Can you work these out from the model? Positions are in its coordinate system, mm. Face numbers are marked on the shaded views. A direction names the side the tool comes from. Give positions to 0.01 mm unless a question says otherwise; leave off trailing zeros. Order: outer loops, then holes, each group sorted by start corner. A loop starts at its lowest first (then second) coordinate and runs counter-clockwise, first axis right, second up. Notation, with made-up numbers: (73, 78) -> (119, 78) arc R10 cw to (119, 95) -> close; hole circle Ø11 at (43.25, -37.75). An arc over 180 degrees is marked (long way). Answer as a JSON object with one key per item and string values.
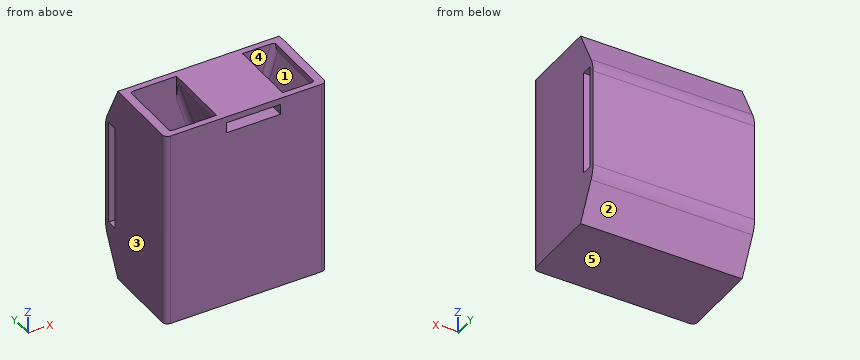
```python
from build123d import *

# Parameters (mm, degrees)
F1_DEPTH  = 3
F2_START  = 3
F2_DEPTH  = 32
F3_START  = 35
F3_DEPTH  = 3
F4_W      = 5
F4_H      = 50
F5_DEPTH  = 76.5907008807
F6_R      = 15
F8_R      = 2.5
F9_R      = 2.5
F7_W      = 25.5907008807
F7_H      = 5
F10_DEPTH = 35


with BuildPart() as f1:
    # F0 (on Front) → F1 (new body)
    with BuildSketch(Plane.XZ):
        Polygon((-29.1335783188, 93.8650974194), (0, 0), (18.3235442432, 0), (47.457122562, 93.8650974194), (43.384812198, 93.8650974194), (43.384812198, 90.8650974194), (16.1134965809, 3), (0.9311313508, 3), (28.2024469679, 90.8650974194), (28.2024469679, 93.8650974194), (-3.0730148629, 93.8650974194), (-3.0730148629, 90.8650974194), (10.9941265459, 45.5423573046), (0, 10.1205238455), (-25.0612679548, 90.8650974194), (-25.0612679548, 93.8650974194), align=None)
        Polygon((-3.0730148629, 93.8650974194), (-25.0612679548, 93.8650974194), (-25.0612679548, 90.8650974194), (0, 10.1205238455), (10.9941265459, 45.5423573046), (-3.0730148629, 90.8650974194), align=None)
        Polygon((43.384812198, 90.8650974194), (43.384812198, 93.8650974194), (28.2024469679, 93.8650974194), (28.2024469679, 90.8650974194), (0.9311313508, 3), (16.1134965809, 3), align=None)
        Polygon((-29.1335783188, 0), (0, 0), (-29.1335783188, 93.8650974194), align=None)
        Polygon((47.457122562, 93.8650974194), (18.3235442432, 0), (47.457122562, 0), align=None)
    extrude(amount=F1_DEPTH)

    # F0 (on Front) → F2 (join)
    with BuildSketch(Plane.XZ.offset(F2_START)):
        Polygon((-29.1335783188, 93.8650974194), (0, 0), (18.3235442432, 0), (47.457122562, 93.8650974194), (43.384812198, 93.8650974194), (43.384812198, 90.8650974194), (16.1134965809, 3), (0.9311313508, 3), (28.2024469679, 90.8650974194), (28.2024469679, 93.8650974194), (-3.0730148629, 93.8650974194), (-3.0730148629, 90.8650974194), (10.9941265459, 45.5423573046), (0, 10.1205238455), (-25.0612679548, 90.8650974194), (-25.0612679548, 93.8650974194), align=None)
        Polygon((-29.1335783188, 0), (0, 0), (-29.1335783188, 93.8650974194), align=None)
        Polygon((47.457122562, 93.8650974194), (18.3235442432, 0), (47.457122562, 0), align=None)
    extrude(amount=F2_DEPTH)

    # F0 (on Front) → F3 (join)
    with BuildSketch(Plane.XZ.offset(F3_START)):
        Polygon((-29.1335783188, 93.8650974194), (0, 0), (18.3235442432, 0), (47.457122562, 93.8650974194), (43.384812198, 93.8650974194), (43.384812198, 90.8650974194), (16.1134965809, 3), (0.9311313508, 3), (28.2024469679, 90.8650974194), (28.2024469679, 93.8650974194), (-3.0730148629, 93.8650974194), (-3.0730148629, 90.8650974194), (10.9941265459, 45.5423573046), (0, 10.1205238455), (-25.0612679548, 90.8650974194), (-25.0612679548, 93.8650974194), align=None)
        Polygon((-3.0730148629, 93.8650974194), (-25.0612679548, 93.8650974194), (-25.0612679548, 90.8650974194), (0, 10.1205238455), (10.9941265459, 45.5423573046), (-3.0730148629, 90.8650974194), align=None)
        Polygon((43.384812198, 90.8650974194), (43.384812198, 93.8650974194), (28.2024469679, 93.8650974194), (28.2024469679, 90.8650974194), (0.9311313508, 3), (16.1134965809, 3), align=None)
        Polygon((-29.1335783188, 0), (0, 0), (-29.1335783188, 93.8650974194), align=None)
        Polygon((47.457122562, 93.8650974194), (18.3235442432, 0), (47.457122562, 0), align=None)
    extrude(amount=F3_DEPTH)

    # F4 (on face) → F5 (join, through all)
    with BuildSketch(Plane.YZ.offset(47.457122562)):
        Polygon((10, 73.8650974194), (0, 93.8650974194), (0, 0), (10, 20), align=None)
        with Locations((5, 48.8650974194)):
            Rectangle(F4_W, F4_H, mode=Mode.SUBTRACT)
    extrude(amount=-F5_DEPTH)

    # F6
    f6_edges = [f1.edges().sort_by_distance(p)[0] for p in [
        (9.161772, 10, 73.865097),
        (9.161772, 10, 20),
    ]]
    fillet(f6_edges, radius=F6_R)

    # F8
    f8_edges = [f1.edges().sort_by_distance(p)[0] for p in [
        (-12.530634, -3, 50.492811),
        (3.960556, -3, 68.203727),
        (3.960556, -35, 68.203727),
        (-12.530634, -35, 50.492811),
        (29.749154, -35, 46.932549),
        (29.749154, -3, 46.932549),
        (14.566789, -3, 46.932549),
        (14.566789, -35, 46.932549),
    ]]
    fillet(f8_edges, radius=F8_R)

    # F9
    f9_edges = [f1.edges().sort_by_distance(p)[0] for p in [
        (-29.133578, -38, 46.932549),
        (47.457123, -38, 46.932549),
    ]]
    fillet(f9_edges, radius=F9_R)

    # F7 (on face) → F10 (cut)
    with BuildSketch(Plane.XZ.offset(38)):
        with Locations((12.6617721216, 88.3650974194)):
            Rectangle(F7_W, F7_H)
    extrude(amount=-F10_DEPTH, mode=Mode.SUBTRACT)


solid = f1.part
```
1. If we mould it in two halves opening along Z, with no side actions, what happens to the marked faces 1, 2 and 3? For each: +Z half, -Z half, draft (parallel to the pull), parting line (faces both ways), or undercut.
Worked answers:
{"face 1": "undercut", "face 2": "-Z half", "face 3": "draft"}
2. If we section it at C-C on z = 72.5: Count the separate pieces of the cut face and the enclosed holes in it, then the cut area to 3 significant figures.
Worked answers:
{"separate pieces": "2", "enclosed holes": "2", "area": "2,100 mm²"}
3. Will these pins go through, and if not, where does the flat tip stop? pin 1 Ø8 at (x, z) = (29.5, 15) entering from +Y; pin 2 Ø1.5 at (x, z) = (9.5, 89) entering from -Y; pin 3 Ø5.5 at (x, y) = (-2.5, 5) entering from +Z.
Worked answers:
{"pin 1": "y = 9.3", "pin 2": "y = -3", "pin 3": "z = 89.37"}
4. Please list where these lines run through material, in increasing order: L1, parallel to Y at x = 1.5, z = 38; L2, parallel to X at y = -34, z = 22; L3, parallel to X at y = -27, z = 20.
Worked answers:
{"L1": "-38 to -35, -3 to 2.5, 7.5 to 10", "L2": "-29.13 to -3.16, 3.69 to 7.35, 21.49 to 47.46", "L3": "-29.13 to -3.07, 3.07 to 6.21, 21.39 to 47.46"}
5. If we section it at B-B on y = 6: Please give me the cut outline in (x, z), then the cut area to 3 significant figures.
Worked answers:
{"outline": "(-29.13, 12) -> (47.46, 12) -> (47.46, 23.87) -> (-29.13, 23.87) -> close; (-29.13, 73.87) -> (47.46, 73.87) -> (47.46, 81.87) -> (-29.13, 81.87) -> close", "area": "1,520 mm²"}
6. If we section it at A-A on y = -14: Please give me the cut outline in (x, z).
Worked answers:
{"outline": "(-29.13, 0) -> (47.46, 0) -> (47.46, 93.87) -> (43.38, 93.87) -> (43.38, 90.87) -> (16.11, 3) -> (0.93, 3) -> (28.2, 90.87) -> (28.2, 93.87) -> (-3.07, 93.87) -> (-3.07, 90.87) -> (10.99, 45.54) -> (0, 10.12) -> (-25.06, 90.87) -> (-25.06, 93.87) -> (-29.13, 93.87) -> close; hole (-0.13, 85.87) -> (25.46, 85.87) -> (25.46, 90.87) -> (-0.13, 90.87) -> close"}
7. For the marked faces 4 and 5, which set-ups out of +Z, -Z, +X, -X, +Y, -Y let a thin tool reach every point of the face, with its end or its side?
Worked answers:
{"face 4": "none", "face 5": "-Z, +X, -X, +Y, -Y"}
